The figure shows three views and two pictorial views of one solid part (mm, origin at its lowest corner). Answer the questions. Coordinates: 2 decimals unless noted, no trailing zeros. Loops run counter-clockwise (first coordinate to the right, second up) from the corner with the lowest first, then second, coordinate; pieces in that order, holes last.
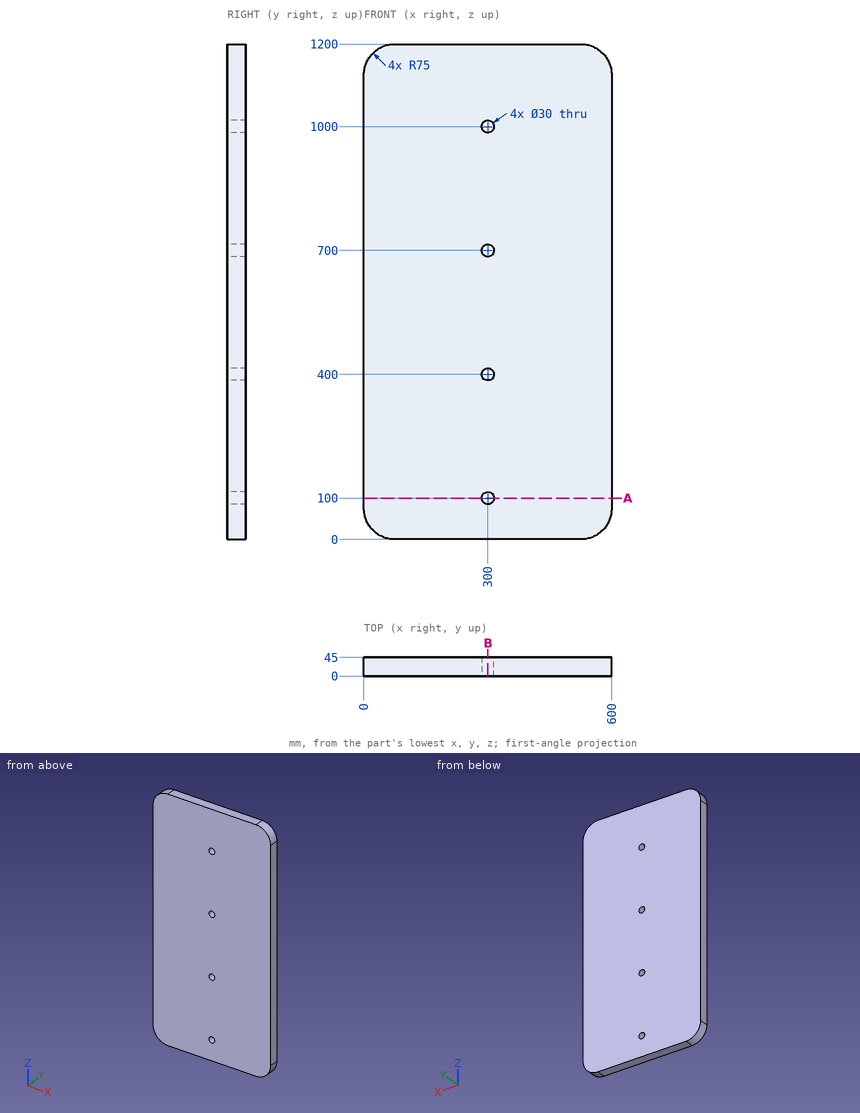
Q1. A cutting plane is placed at B-B (x = 300). Give the vertices of the cut face in (y, z).
Findings below:
outline: (0, 0) - (45, 0) - (45, 85) - (0, 85) - close; (0, 115) - (45, 115) - (45, 385) - (0, 385) - close; (0, 415) - (45, 415) - (45, 685) - (0, 685) - close; (0, 715) - (45, 715) - (45, 985) - (0, 985) - close; (0, 1015) - (45, 1015) - (45, 1200) - (0, 1200) - close
Q2. A cutting plane is placed at A-A (z = 100). Give the vertices of the cut face in (x, y), then the cut area to 4 significant figures.
Findings below:
outline: (0, 0) - (285, 0) - (285, 45) - (0, 45) - close; (315, 0) - (600, 0) - (600, 45) - (315, 45) - close
area: 25,650 mm2
Q3. Straight lines are drawn through the part: probe 1 along Z at (x, y) = (300, 20); probe 2 along X at (y, z) = (26, 1000); probe 3 along X at (y, z) = (18.5, 709). For each, find the intervals that lie inside material, in ascending order.
Findings below:
probe 1: z = 0 to 85, 115 to 385, 415 to 685, 715 to 985, 1015 to 1200
probe 2: x = 0 to 285, 315 to 600
probe 3: x = 0 to 288, 312 to 600
